The listing builds one solid part. Answer for the finished solid, in the listing's coordinates (mm). A direction names the side the tool comes from. Give positions to 0.01 mm unless a question says otherwise; leave off trailing zeros. Loops run counter-clockwise (first coordinate to the right, second up) from the corner with the lowest first, then second, coordinate; pieces in that order, holes last. Notation, with made-up numbers: (36.25, 86.5) -> (59.25, 86.5) arc R35 cw to (59.25, 123.5) -> close; hole circle Ø2 at (-16.75, -32). An arc over 180 degrees is marked (long way). One line per question, with ' | ' between items. Start each with the question number.
from build123d import *

# Parameters (mm, degrees)
SKETCH1_W           = 482.6
SKETCH1_H           = 50.8
BOSS_EXTRUDE1_DEPTH = 76.2
CUT_EXTRUDE2_DEPTH  = 49.022
SKETCH3_W           = 482.6
SKETCH3_H           = 16.002
CUT_EXTRUDE3_DEPTH  = 31.75
SKETCH4_W           = 482.6
SKETCH4_H           = 15.748
CUT_EXTRUDE4_DEPTH  = 12.7
SHELL2_START        = -23.622
SHELL2_OUTLINE_W    = 479.044
SHELL2_OUTLINE_H    = 14.224
SHELL2_DEPTH        = 47.244
SKETCH5_W           = 1.778
SKETCH5_H           = 17.272
BOSS_EXTRUDE2_DEPTH = 44.45
FILLET1_R           = 2.54
SKETCH6_R           = 3.81
CUT_EXTRUDE5_DEPTH  = 44.45


# Read off the part's stored shape, not the designer's step: Shell2
with BuildPart() as part:
    # Sketch1 → Boss-Extrude1 (new body)
    with BuildSketch(Plane.XY):
        Rectangle(SKETCH1_W, SKETCH1_H)
    extrude(amount=BOSS_EXTRUDE1_DEPTH)

    # Sketch2 → Cut-Extrude2 (cut)
    with BuildSketch(Plane(origin=(0, 25.4, 0), x_dir=(1, 0, 0), z_dir=(0, 1, 0))):
        Polygon((241.3, -16.002), (-241.3, -16.002), (-241.3, -38.1), (-241.3, -60.198), (241.3, -60.198), align=None)
    extrude(amount=-CUT_EXTRUDE2_DEPTH, mode=Mode.SUBTRACT)

    # Sketch3 → Cut-Extrude3 (cut)
    with BuildSketch(Plane(origin=(0, 25.4, 0), x_dir=(1, 0, 0), z_dir=(0, 1, 0))):
        with Locations((0, -68.199)):
            Rectangle(SKETCH3_W, SKETCH3_H)
    extrude(amount=-CUT_EXTRUDE3_DEPTH, mode=Mode.SUBTRACT)

    # Sketch4 → Cut-Extrude4 (cut)
    with BuildSketch(Plane.XY.offset(76.2)):
        with Locations((0, -17.526)):
            Rectangle(SKETCH4_W, SKETCH4_H)
    extrude(amount=-CUT_EXTRUDE4_DEPTH, mode=Mode.SUBTRACT)

    # Shell2 outline → Shell2 (cut)
    with BuildSketch(Plane(origin=(0, 0, 0), x_dir=(1, 0, 0), z_dir=(0, 1, 0)).offset(SHELL2_START)):
        with Locations((0, -8.89)):
            Rectangle(SHELL2_OUTLINE_W, SHELL2_OUTLINE_H)
    extrude(amount=SHELL2_DEPTH, mode=Mode.SUBTRACT)

    # Sketch5 → Boss-Extrude2 (add)
    with BuildSketch(Plane(origin=(0, 0, 60.198), x_dir=(-1, 0, 0), z_dir=(0, 0, -1))):
        with Locations((240.411, -14.986)):
            Rectangle(SKETCH5_W, SKETCH5_H)
        with Locations((-240.411, -14.986)):
            Rectangle(SKETCH5_W, SKETCH5_H)
    extrude(amount=BOSS_EXTRUDE2_DEPTH)

    # Fillet1
    fillet1_edges = [part.edges().sort_by_distance(p)[0] for p in [
        (0, -25.4, 0),
        (0, -25.4, 63.5),
        (0, 25.4, 0),
        (0, -6.35, 60.198),
    ]]
    fillet(fillet1_edges, radius=FILLET1_R)

    # Sketch6 → Cut-Extrude5 (cut)
    with BuildSketch(Plane(origin=(0, -23.622, 0), x_dir=(1, 0, 0), z_dir=(0, 1, 0))):
        with Locations(Location((-132.842, -14.478, 0), (0, 0, 270))):
            Circle(SKETCH6_R)
        with Locations(Location((132.842, -14.478, 0), (0, 0, 270))):
            Circle(SKETCH6_R)
    extrude(amount=-CUT_EXTRUDE5_DEPTH, mode=Mode.SUBTRACT)


solid = part.part
1. Straight lines are drawn through the part: L1, parallel to Z at x = -122.5, y = -13.5; L2, parallel to Y at x = -104, z = 8; L3, parallel to X at y = -16, z = 53. For each, find the intervals that lie inside material, in ascending order.
2. The part is cut by section B-B (x = -47). Write down the section's boundary in (y, z).
3. Each of these flat-tipped pins is pushed along its axis until it touches: pin 1 Ø12 at (x, z) = (-132.842, 14.478) entering from -Y; pin 2 Ø6 at (x, z) = (-134.5, 54) entering from +Y; pin 3 Ø3 at (x, z) = (-109, 63.5) entering from -Y; pin 4 Ø4 at (x, z) = (22.5, 61) entering from +Y. Where does it stop, or does it pass through?
4. The part is cut by section A-A (z = 28.5). Write down the section's boundary in (x, y), plus the area to 3 significant figures.
5. Determine the mould class of faces 1 (the flat face through (-239.522, -11, 26)), 2 (the flat face through (-3, 0, 0)), 3 (the flat face through (241.3, -12, 29)) for opening direction X: released by +X, released by -X, zero draft, split by the parting line, or undercut.
6. For faces 4 (the flat face through (1, -6.35, 71)), 5 (the flat face through (-3, -23.622, 31)), 6 (the cylindrical face through (-136.56, -24.5, 13.65)), determine the directions among +Z, -Z, +X, -X, +Y, -Y from which every point of the face is accessible in a straight line to the end or side of a thin tool.
7. The part is cut by section C-C (y = -0.5). Write down the section's boundary in (x, z).
Check sheet entries:
1) L1: z = 0 to 1.78, 60.2 to 63.5 | L2: y = -25.4 to -23.62, 23.62 to 25.4 | L3: x = -241.3 to -239.52, 239.52 to 241.3
2) outline: (-25.4, 2.54) arc R2.54 ccw to (-22.86, 0) -> (22.86, 0) arc R2.54 ccw to (25.4, 2.54) -> (25.4, 16) -> (23.62, 16) -> (23.62, 1.78) -> (-23.62, 1.78) -> (-23.62, 60.2) -> (-8.89, 60.2) arc R2.54 ccw to (-6.35, 62.74) -> (-6.35, 76.2) -> (-9.65, 76.2) -> (-9.65, 63.5) -> (-22.86, 63.5) arc R2.54 ccw to (-25.4, 60.96) -> close
3) pin 1: stops at y = -25.4 | pin 2: stops at y = -23.62 | pin 3: stops at y = -25.18 | pin 4: stops at y = -6.35
4) outline: (-241.3, -25.4) -> (241.3, -25.4) -> (241.3, -6.35) -> (239.52, -6.35) -> (239.52, -23.62) -> (-239.52, -23.62) -> (-239.52, -6.35) -> (-241.3, -6.35) -> close | area: 919 mm^2
5) face 1: undercut | face 2: zero draft | face 3: released by +X
6) face 4: +Z, +X, -X, +Y | face 5: none | face 6: -Y
7) outline: (-241.3, 0) -> (241.3, 0) -> (241.3, 16) -> (239.52, 16) -> (239.52, 1.78) -> (-239.52, 1.78) -> (-239.52, 16) -> (-241.3, 16) -> close
